Read the model definition and answer for the solid it produces. Units are mm, in the model's axes. A direction names the side the tool comes from. Give positions to 0.01 mm unless a question says otherwise; leave off trailing zeros. Order: outer loops, then holes, each group sorted by start corner. A loop starts at its lowest first (then second) coordinate and runs counter-clockwise, first axis right, second up.
```python
from build123d import *

# Parameters (mm, degrees)
IZIM3_R                     = 12.5
IZIM3_R_2                   = 8
Y_KSEKLIK_EKSTR_ZYON1_DEPTH = 12
IZIM3_3_R                   = 8
Y_KSEKLIK_EKSTR_ZYON2_DEPTH = 32
PAH1_SIZE                   = 1
KES_EKSTR_ZYON1_DEPTH       = 48.418350878
KES_EKSTR_ZYON1_DEPTH_BACK  = 4
IZIM4_W                     = 2
IZIM4_H                     = 25


with BuildPart() as part:
    # izim3 → Y_kseklik-Ekstr_zyon1 (new body)
    # profile 1 of 2: a face of its own
    with BuildSketch(Plane(origin=(0, 0, 0), x_dir=(1, 0, 0), z_dir=(0, 1, 0))):
        with Locations(Location((0, 0, 0), (0, 0, 270))):
            Circle(IZIM3_R)
        Circle(IZIM3_R_2, mode=Mode.SUBTRACT)
    # profile 2 of 2: a face of its own
    with BuildSketch(Plane(origin=(0, 0, 0), x_dir=(1, 0, 0), z_dir=(0, 1, 0))):
        Circle(IZIM3_R_2)
    extrude(amount=Y_KSEKLIK_EKSTR_ZYON1_DEPTH)

    # izim3_3 → Y_kseklik-Ekstr_zyon2 (add)
    with BuildSketch(Plane(origin=(0, 0, 0), x_dir=(1, 0, 0), z_dir=(0, 1, 0))):
        with Locations(Location((0, 0, 0), (0, 0, 270))):
            Circle(IZIM3_3_R)
    extrude(amount=-Y_KSEKLIK_EKSTR_ZYON2_DEPTH)

    # Pah1
    pah1_edges = [part.edges().sort_by_distance(p)[0] for p in [
        (0, -32, -8),
    ]]
    chamfer(pah1_edges, length=PAH1_SIZE)

    # izim4 → Kes-Ekstr_zyon1 (cut, two sides: drawn at the far end of the back side and taken through both)
    with BuildSketch(Plane(origin=(0, 12, 0), x_dir=(1, 0, 0), z_dir=(0, 1, 0)).offset(-KES_EKSTR_ZYON1_DEPTH_BACK)):
        Rectangle(IZIM4_W, IZIM4_H)
    extrude(amount=KES_EKSTR_ZYON1_DEPTH + KES_EKSTR_ZYON1_DEPTH_BACK, mode=Mode.SUBTRACT)


solid = part.part
```
1) For a pull along X with two mould halves and no side action, classify faces 1 (the face through (-0.2, 0, 8.2)), 2 (the face through (1, 10, 0)), 3 (the face through (3.755, 5.916, 11.923)) as released by +X, released by -X, zero draft, split by the parting line, or undercut.
Final values:
face 1: zero draft
face 2: undercut
face 3: split by the parting line
2) Consider L1, parallel to Z at x = -0.25, y = -29.5; L2, parallel to Y at x = 10.5, z = 5.5; L3, parallel to Y at x = -0.75, z = -6.75. Determine where each line is inside the solid, lowest interval first.
Final values:
L1: z = -8 to 8
L2: y = 0 to 12
L3: y = -32 to 8
3) The part is cut by section A-A on x = 0. Determine the outline of the cut face in (y, z).
Final values:
outline: (-32, -7) - (-31, -8) - (0, -8) - (0, -12.5) - (8, -12.5) - (8, 12.5) - (0, 12.5) - (0, 8) - (-31, 8) - (-32, 7) - close
4) A tool of negligible diameter and unlimited length cuts with its end or side. For faces 4 (the face through (-7.81, -15.28, -1.73)), 5 (the face through (6, 12, 0)), 6 (the face through (0, 8, 0)), from which of +Z, -Z, +X, -X, +Y, -Y can it reach the whole face along a straight path? Write none if from no direction.
Final values:
face 4: -Y
face 5: +Z, -Z, +X, -X, +Y
face 6: +Z, -Z, +Y
5) The part is cut by section D-D on y = 5. Determine the outline of the cut face in (x, z).
Final values:
outline: circle Ø25 at (0, 0)
6) The part is cut by section B-B on z = 0. Determine the outline of the cut face in (x, y), and give its area (3 significant figures).
Final values:
outline: (-12.5, 0) - (-8, 0) - (-8, -31) - (-7, -32) - (7, -32) - (8, -31) - (8, 0) - (12.5, 0) - (12.5, 12) - (1, 12) - (1, 8) - (-1, 8) - (-1, 12) - (-12.5, 12) - close
area: 803 mm2
7) The part is cut by section C-C on y = -23. Determine the outline of the cut face in (x, z), and give its area (3 significant figures).
Final values:
outline: circle Ø16 at (0, 0)
area: 201 mm2
8) Given pin 1 (2 mm diameter, centred on x = -1, y = -24, fed in from -Z); pin 2 (12 mm diameter, centred on x = 7, y = -6.5, fed in from +Z); pin 3 (3 mm diameter, centred on y = 9, z = -3.5, fed in from -X), each flat-ended and moving along its own axis, determine where each tip first touches the part or whether it passes through.
Final values:
pin 1: stops at z = -8
pin 2: stops at z = 7.94
pin 3: stops at x = -12.34
